Could you check a few things on this model? Use its own coordinates, in mm. A direction names the side the tool comes from. Coordinates: 2 decimals unless noted, no trailing zeros. Write each loop counter-clockwise with the first axis right and the second up, starting at its lowest first coordinate (ties: lowest second). Pieces come first, ordered by that corner, then holes.
```python
from build123d import *

# Parameters (mm, degrees)
BOSS_EXTRUDE1_DEPTH      = 30
BOSS_EXTRUDE1_DEPTH_BACK = 30
SKETCH1_R                = 10
BOSS_EXTRUDE2_DEPTH      = 30
BOSS_EXTRUDE2_DEPTH_BACK = 30
SKETCH2_R                = 10


with BuildPart() as part:
    # Sketch1 → Boss-Extrude1 (new, two sides: drawn at the far end of the back side and taken through both)
    with BuildSketch(Plane.XY.offset(-BOSS_EXTRUDE1_DEPTH_BACK)):
        Circle(SKETCH1_R)
    extrude(amount=BOSS_EXTRUDE1_DEPTH + BOSS_EXTRUDE1_DEPTH_BACK)

    # Sketch2 → Boss-Extrude2 (add, two sides: drawn at the far end of the back side and taken through both)
    with BuildSketch(Plane(origin=(0, 0, 0), x_dir=(0, 0, -1), z_dir=(1, 0, 0)).offset(-BOSS_EXTRUDE2_DEPTH_BACK)):
        Circle(SKETCH2_R)
    extrude(amount=BOSS_EXTRUDE2_DEPTH + BOSS_EXTRUDE2_DEPTH_BACK)


solid = part.part
```
1. On a 3-axis mill with a long thin cutter (end or side, diameter ignored), from which of +Z, -Z, +X, -X, +Y, -Y can I reach the whole of each face in a straight line? I mean faces 3 (the face through (18, 0, 10)), 4 (the face through (-19, 0, 10)), 5 (the face through (-10, 0, -19)). Say none if no direction works.
Verdict:
face 3: +X
face 4: -X
face 5: -Z
2. I want a section at C-C on z = -7. Please give me the cut outline in (x, y), plus the area to 3 significant figures.
Verdict:
outline: (-30, -7.14) - (-7, -7.14) arc R10 ccw to (7, -7.14) - (30, -7.14) - (30, 7.14) - (7, 7.14) arc R10 ccw to (-7, 7.14) - (-30, 7.14) - close
area: 912 mm2
3. I want a section at D-D on y = 0.75. Please give me the cut outline in (x, z), plus the area to 3 significant figures.
Verdict:
outline: (-30, -9.97) - (-9.97, -9.97) - (-9.97, -30) - (9.97, -30) - (9.97, -9.97) - (30, -9.97) - (30, 9.97) - (9.97, 9.97) - (9.97, 30) - (-9.97, 30) - (-9.97, 9.97) - (-30, 9.97) - close
area: 2,000 mm2
4. For pin 1 (10 mm diameter, centred on x = 14, z = -16.5, fed in from -Y); pin 2 (3 mm diameter, centred on x = 6, z = 17.5, fed in from -Y); pin 3 (2 mm diameter, centred on x = -6, z = 19.5, fed in from -Y); pin 4 (10 mm diameter, centred on y = -3.5, z = -14.5, fed in from +X), each with a flat end and sliding along its axis, tell me the tip position at first contact or that it passes through.
Verdict:
pin 1: stops at y = -4.36
pin 2: stops at y = -8.93
pin 3: stops at y = -8.66
pin 4: stops at x = 30
5. If we mould it in two halves opening along Y, with no side actions, what happens to faces 1 (the face through (-10, 0, 18)), 2 (the face through (0, 0, 30))? For each: pulls with the +Y half, pulls with the -Y half, needs draft (parallel to the pull), parting line crosses it, or undercut.
Verdict:
face 1: parting line crosses it
face 2: needs draft
6. I want a section at A-A on x = 4. Please give me the cut outline in (y, z).
Verdict:
outline: (-9.17, -30) - (9.17, -30) - (9.17, -4) arc R10 ccw to (9.17, 4) - (9.17, 30) - (-9.17, 30) - (-9.17, 4) arc R10 ccw to (-9.17, -4) - close
7. I want a section at B-B on y = -2.5. Please give me the cut outline in (x, z), plus the area to 3 significant figures.
Verdict:
outline: (-30, -9.68) - (-9.68, -9.68) - (-9.68, -30) - (9.68, -30) - (9.68, -9.68) - (30, -9.68) - (30, 9.68) - (9.68, 9.68) - (9.68, 30) - (-9.68, 30) - (-9.68, 9.68) - (-30, 9.68) - close
area: 1,950 mm2
8. Please list where these lines run through material, in increasing order: line 1 along X through (y, z) = (0, -26); line 2 along X through (y, z) = (-4, 23).
Verdict:
line 1: x = -10 to 10
line 2: x = -9.17 to 9.17
